The listing builds one solid part. Answer for the finished solid, in the listing's coordinates (mm). A direction names the side the tool comes from. Coordinates: 2 decimals unless noted, no trailing zeros. Order: outer loops, then holes, each group sorted by start corner. A loop starts at its lowest first (then second) coordinate and runs counter-clockwise, first axis right, second up. Notation, with made-up numbers: (7, -33.75) -> (36, -33.75) arc R20 ccw to (36, -16.75) -> close; hole circle Ø4 at (44, 85). An arc over 180 degrees is marked (long way). Return JSON: item names as keys, results as strings.
```python
from build123d import *

# Parameters (mm, degrees)
SKETCH_1_W          = 40
SKETCH_1_H          = 40
SKETCH_1_R          = 2.25
EXTRUDE_1_DEPTH     = 1.6
EXTRUDE_2_DEPTH     = 6.5
SKETCH_3_R          = 4
CUT_EXTRUDE_1_DEPTH = 30.421250823


with BuildPart() as part:
    # ｽｹｯﾁ1 → ﾎﾞｽ - 押し出し1 (new body)
    with BuildSketch(Plane(origin=(0, 0, 0), x_dir=(1, 0, 0), z_dir=(0, 1, 0))):
        Rectangle(SKETCH_1_W, SKETCH_1_H)
        with Locations(Location((-12, 12, 0), (0, 0, 270))):
            Circle(SKETCH_1_R, mode=Mode.SUBTRACT)
        with Locations(Location((12, 12, 0), (0, 0, 270))):
            Circle(SKETCH_1_R, mode=Mode.SUBTRACT)
        with Locations(Location((-12, -12, 0), (0, 0, 270))):
            Circle(SKETCH_1_R, mode=Mode.SUBTRACT)
        with Locations(Location((12, -12, 0), (0, 0, 270))):
            Circle(SKETCH_1_R, mode=Mode.SUBTRACT)
    extrude(amount=EXTRUDE_1_DEPTH)

    # ｽｹｯﾁ2 → ﾎﾞｽ - 押し出し2 (add)
    with BuildSketch(Plane(origin=(0, 1.6, 0), x_dir=(1, 0, 0), z_dir=(0, 1, 0))):
        Polygon((0, 7.5), (6.5, 3.751666445), (6.5, -3.751666445), (0, -7.5), (-6.5, -3.751666445), (-6.5, 3.751666445), align=None)
    extrude(amount=EXTRUDE_2_DEPTH)

    # ｽｹｯﾁ3 → ｶｯﾄ - 押し出し1 (cut, through all)
    with BuildSketch(Plane(origin=(0, 8.1, 0), x_dir=(1, 0, 0), z_dir=(0, 1, 0))):
        with Locations(Location((0, 0, 0), (0, 0, 270))):
            Circle(SKETCH_3_R)
    extrude(amount=-CUT_EXTRUDE_1_DEPTH, mode=Mode.SUBTRACT)


solid = part.part
```
Item 1: Find the intervals of material crossed by probe 1 along X at (y, z) = (0.4, 12); probe 2 along Y at (x, z) = (-1.5, -14); probe 3 along Z at (x, y) = (-10, 1), in increasing order.
Answer list:
{"probe 1": "-20 to -14.25, -9.75 to 9.75, 14.25 to 20", "probe 2": "0 to 1.6", "probe 3": "-20 to -13.03, -10.97 to 10.97, 13.03 to 20"}
Item 2: The part is cut by section B-B on x = 12. Determine the outline of the cut face in (y, z).
Answer list:
{"outline": "(0, -20) -> (1.6, -20) -> (1.6, -14.25) -> (0, -14.25) -> close; (0, -9.75) -> (1.6, -9.75) -> (1.6, 9.75) -> (0, 9.75) -> close; (0, 14.25) -> (1.6, 14.25) -> (1.6, 20) -> (0, 20) -> close"}
Item 3: The part is cut by section D-D on x = -16. Determine the outline of the cut face in (y, z).
Answer list:
{"outline": "(0, -20) -> (1.6, -20) -> (1.6, 20) -> (0, 20) -> close"}
Item 4: Flat-ended cylindrical pins translate along their axes: pin 1 (1.5 mm diameter, centred on y = 3.5, z = -10, fed in from +X); pin 2 (3 mm diameter, centred on y = 5.5, z = 0.5, fed in from +X); pin 3 (3 mm diameter, centred on y = 4.5, z = -3.5, fed in from -X). Find the tip coordinate at first contact, or state that the pin passes through.
Answer list:
{"pin 1": "through", "pin 2": "x = 6.5", "pin 3": "x = -6.5"}
Item 5: The part is cut by section C-C on y = 6. Determine the outline of the cut face in (x, z), plus the area to 3 significant figures.
Answer list:
{"outline": "(-6.5, -3.75) -> (0, -7.5) -> (6.5, -3.75) -> (6.5, 3.75) -> (0, 7.5) -> (-6.5, 3.75) -> close; hole circle Ø8 at (0, 0)", "area": "96.0 mm2"}
Item 6: The part is cut by section A-A on z = -12. Determine the outline of the cut face in (x, y).
Answer list:
{"outline": "(-20, 0) -> (-14.25, 0) -> (-14.25, 1.6) -> (-20, 1.6) -> close; (-9.75, 0) -> (9.75, 0) -> (9.75, 1.6) -> (-9.75, 1.6) -> close; (14.25, 0) -> (20, 0) -> (20, 1.6) -> (14.25, 1.6) -> close"}
Item 7: Determine the mould class of faces 1 (the cylindrical face through (13.52, 0.79, -13.66)), 2 (the flat face through (-3.295, 4.804, -5.6)), 3 (the flat face through (-5, 0, 0)) for opening direction Z: pulls with the +Z half, pulls with the -Z half, needs draft (parallel to the pull), parting line crosses it, or undercut.
Answer list:
{"face 1": "undercut", "face 2": "pulls with the -Z half", "face 3": "needs draft"}
Item 8: Which of the six approach directions +Z, -Z, +X, -X, +Y, -Y give full straight-line access (tool end or side, diameter ignored) to faces 4 (the flat face through (-6.5, 5, 0)), 5 (the flat face through (6.5, 5, 0)), 6 (the flat face through (0, 1.6, -9))?
Answer list:
{"face 4": "+Z, -Z, -X, +Y", "face 5": "+Z, -Z, +X, +Y", "face 6": "+Y"}
